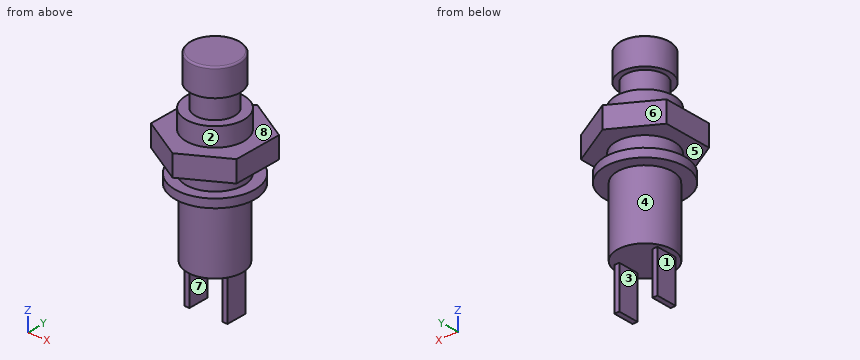
```python
from build123d import *

# Parameters (mm, degrees)
SKETCH1_R        = 4.675
COLLAR_DEPTH     = 1
SKETCH2_R        = 3.4
FRONT_BODY_DEPTH = 6.7
SKETCH4_R        = 2.3
SHAFT_DEPTH      = 2.6
SKETCH5_R        = 2.93
KNOB_DEPTH       = 3.2
KNOB_FILLET_R    = 0.2
SKETCH3_R        = 3.25
REAR_BODY_DEPTH  = 9
SKETCH6_W        = 0.6
SKETCH6_H        = 2.5
PINS_DEPTH       = 5
NUT_DEPTH        = 2.5


with BuildPart() as part:
    # Sketch1 → Collar (new body)
    with BuildSketch(Plane.XY):
        Circle(SKETCH1_R)
    extrude(amount=-COLLAR_DEPTH)

    # Sketch2 → Front Body (add)
    with BuildSketch(Plane.XY):
        Circle(SKETCH2_R)
    extrude(amount=FRONT_BODY_DEPTH)

    # Sketch4 → Shaft (add)
    with BuildSketch(Plane.XY.offset(6.7)):
        Circle(SKETCH4_R)
    extrude(amount=SHAFT_DEPTH)

    # Sketch5 → Knob (add)
    with BuildSketch(Plane.XY.offset(9.3)):
        Circle(SKETCH5_R)
    extrude(amount=KNOB_DEPTH)

    # Knob Fillet
    knob_fillet_edges = [part.edges().sort_by_distance(p)[0] for p in [
        (-2.93, 0, 12.5),
    ]]
    fillet(knob_fillet_edges, radius=KNOB_FILLET_R)

    # Sketch3 → Rear Body (add)
    with BuildSketch(Plane.XY):
        Circle(SKETCH3_R)
    extrude(amount=-REAR_BODY_DEPTH)

    # Sketch6 → Pins (add)
    with BuildSketch(Plane(origin=(0, 0, -9), x_dir=(-1, 0, 0), z_dir=(0, 0, -1))):
        with Locations((-2.25, 0)):
            Rectangle(SKETCH6_W, SKETCH6_H)
        with Locations((2.25, 0)):
            Rectangle(SKETCH6_W, SKETCH6_H)
    extrude(amount=PINS_DEPTH)

    # Sketch7 → Nut (add)
    with BuildSketch(Plane.XY.offset(2)):
        Polygon((0, 5.831237719), (-5.05, 2.915618859), (-5.05, -2.915618859), (0, -5.831237719), (5.05, -2.915618859), (5.05, 2.915618859), align=None)
    extrude(amount=NUT_DEPTH)


solid = part.part
```
Geometry check sheet. Reference: the model listing, model coordinates, mm. Face numbers are marked on the shaded views. A direction names the side the tool comes from. Coordinates: 2 decimals unless noted, no trailing zeros. Write each loop counter-clockwise with the first axis right and the second up, starting at its lowest first coordinate (ties: lowest second). Pieces come first, ordered by that corner, then holes. Notation, with made-up numbers: M -10.5,-15 L 18.5,-15 A18 cw 18.5,9 Z; hole C 54.5,65 d5. An arc over 180 degrees is marked long. Use one line per item in the form item = value. Start each with the question number.
1) Set-up check for the marked faces 1, 2, 3, 4 and 5: record each of +Z, -Z, +X, -X, +Y, -Y from which the full face is reachable in a straight line by a thin tool's end or side.
2) Section check D-D on z = 7. Enter the section's corners in (x, y), and give its area (3 significant figures).
3) Thickness scan on probe 1 along Z at (x, y) = (-2, 1.5); probe 2 along Z at (x, y) = (3.5, 2); probe 3 along Z at (x, y) = (-4.5, -3). Record the ranges inside material, lowest first. Write a range as from..to.
4) Release check for a two-part mould opening along X. For the marked faces 6, 7 and 8 record: pulls with the +X half, pulls with the -X half, needs draft (parallel to the pull), parting line crosses it, or undercut.
5) Section check B-B on z = 4. Enter the section's corners in (x, y).
6) Go/stop test with flat-tipped pins: pin 1 Ø2 at (y, z) = (-0.5, -11.5) entering from -X; pin 2 Ø5 at (y, z) = (-4, -1) entering from +X; pin 3 Ø1 at (x, y) = (0.5, -2) entering from -Z; pin 4 Ø5 at (x, y) = (1, -1.5) entering from -Z. Record where each tip stops, or that it passes through.
7) Section check A-A on z = -9.5. Enter the section's corners in (x, y), and give its area (3 significant figures).
8) Section check C-C on z = 10.25. Enter the section's corners in (x, y), and give its area (3 significant figures).
Responses:
q1.face_1 = -Z, -X, +Y, -Y
q1.face_2 = +Z
q1.face_3 = -Z, +Y, -Y
q1.face_4 = -Z
q1.face_5 = none
q2.outline = C 0,0 d4.6
q2.area = 16.6 mm2
q3.probe_1 = -9..6.7, 9.3..12.5
q3.probe_2 = -1..0, 2..4.5
q3.probe_3 = 2..4.5
q4.face_6 = pulls with the -X half
q4.face_7 = undercut
q4.face_8 = needs draft
q5.outline = M -5.05,-2.92 L 0,-5.83 L 5.05,-2.92 L 5.05,2.92 L 0,5.83 L -5.05,2.92 Z
q6.pin_1 = -2.55
q6.pin_2 = 4.43
q6.pin_3 = -9
q6.pin_4 = -14
q7.outline = M -2.55,-1.25 L -1.95,-1.25 L -1.95,1.25 L -2.55,1.25 Z; M 1.95,-1.25 L 2.55,-1.25 L 2.55,1.25 L 1.95,1.25 Z
q7.area = 3.00 mm2
q8.outline = C 0,0 d5.86
q8.area = 27.0 mm2
